Could you check a few things on this model? Use its own coordinates, in mm. A direction names the side the tool comes from. Coordinates: 2 decimals unless noted, no trailing zeros. Order: outer loops, then holes, each group sorted by start corner. A loop starts at its lowest first (then second) coordinate and runs counter-clockwise, first axis right, second up. Notation, with made-up numbers: (9, 71.5) -> (64, 71.5) arc R24 cw to (64, 109.5) -> close; hole circle Ø2 at (-18.5, 9). An arc over 180 degrees is marked (long way). Use a Markdown table: item, result. Add a question column.
1) If we section it at B-B (x = 54): Write out the boundary of the cut face in (y, z).
2) If we section it at D-D (z = -1): Write out the boundary of the cut face in (x, y).
3) If we section it at A-A (z = -6): Give the number of separate pieces and of enclosed holes in the cut face, plus the area to 3 significant figures.
4) Thinking about a two-plate mould opening in X: for faces 5 (the flat face through (43, 6, 0)), 6 (the cylindrical face through (26.11, 2.46, -7.34)), 7 (the cylindrical face through (21.804, 15.944, -6.488)), 8 (the flat face through (76, 6, -8)), which applies, +X half, -X half, draft (parallel to the pull), parting line (faces both ways), or undercut?
5) Which directions (+Z, -Z, +X, -X, +Y, -Y) give clear straight access to the entire face, cutting with the end or side of a thin tool? Please do faces 1 (the cylindrical face through (62.004, 15.944, -4.962)), 2 (the flat face through (24, 5, -8)), 3 (the cylindrical face through (59, 6, -11)), 4 (the cylindrical face through (22.513, 12.395, -5.805)).
6) Will these pins go through, and if not, where does the flat tip stop? pin 1 Ø4.5 at (x, z) = (64, -6) entering from -Y; pin 2 Ø3 at (x, y) = (53, 4.5) entering from -Z; pin 3 Ø3 at (x, z) = (59, -10) entering from +Y.
7) If we section it at C-C (y = 15): Write out the boundary of the cut face in (x, z).
8) If I drill on L1, parallel to X at y = 14.5, z = -6; L2, parallel to Y at x = 54, z = -9.75; L3, parallel to Y at x = 75.5, z = -1.5, over which ranges is the centre line in solid material (lowest first)? Write a range as [from, to].
```python
from build123d import *

# Parameters (mm, degrees)
BOSS_EXTRUDE1_DEPTH = 12
SKETCH2_R           = 2.5
CUT_EXTRUDE1_DEPTH  = 5
SKETCH3_R           = 1.5
CUT_EXTRUDE2_DEPTH  = 90.089842294
SKETCH4_R           = 2.25
SKETCH4_R_2         = 1.5
BOSS_EXTRUDE2_DEPTH = 8
SKETCH5_R           = 5
CUT_EXTRUDE3_DEPTH  = 3
SKETCH6_R           = 1.5
CUT_EXTRUDE4_DEPTH  = 91.691785736


with BuildPart() as part:
    # Sketch1 → Boss-Extrude1 (new body)
    with BuildSketch(Plane(origin=(0, 0, 0), x_dir=(1, 0, 0), z_dir=(0, 1, 0))):
        Polygon((0, 0), (88, 0), (88, 4), (64, 12), (24, 12), (0, 4), align=None)
    extrude(amount=BOSS_EXTRUDE1_DEPTH)

    # Sketch2 → Cut-Extrude1 (cut)
    with BuildSketch(Plane(origin=(0, 0, 0), x_dir=(-1, 0, 0), z_dir=(0, -1, 0))):
        with Locations(Location((-24, 6, 0), (0, 0, 90))):
            Circle(SKETCH2_R)
        with Locations(Location((-64, 6, 0), (0, 0, 90))):
            Circle(SKETCH2_R)
    extrude(amount=-CUT_EXTRUDE1_DEPTH, mode=Mode.SUBTRACT)

    # Sketch3 → Cut-Extrude2 (cut, through all)
    with BuildSketch(Plane(origin=(0, 5, 0), x_dir=(-1, 0, 0), z_dir=(0, -1, 0))):
        with Locations(Location((-24, 6, 0), (0, 0, 90))):
            Circle(SKETCH3_R)
        with Locations(Location((-64, 6, 0), (0, 0, 90))):
            Circle(SKETCH3_R)
    extrude(amount=-CUT_EXTRUDE2_DEPTH, mode=Mode.SUBTRACT)

    # Sketch4 → Boss-Extrude2 (add)
    with BuildSketch(Plane(origin=(0, 12, 0), x_dir=(1, 0, 0), z_dir=(0, 1, 0))):
        with Locations(Location((24, 6, 0), (0, 0, 270))):
            Circle(SKETCH4_R)
        with Locations(Location((24, 6, 0), (0, 0, 90))):
            Circle(SKETCH4_R_2, mode=Mode.SUBTRACT)
        with Locations(Location((64, 6, 0), (0, 0, 270))):
            Circle(SKETCH4_R)
        with Locations(Location((64, 6, 0), (0, 0, 90))):
            Circle(SKETCH4_R_2, mode=Mode.SUBTRACT)
    extrude(amount=BOSS_EXTRUDE2_DEPTH)

    # Sketch5 → Cut-Extrude3 (cut)
    with BuildSketch(Plane(origin=(0, 0, -12), x_dir=(-1, 0, 0), z_dir=(0, 0, -1))):
        with Locations((-54, 6)):
            Circle(SKETCH5_R)
    extrude(amount=-CUT_EXTRUDE3_DEPTH, mode=Mode.SUBTRACT)

    # Sketch6 → Cut-Extrude4 (cut, through all)
    with BuildSketch(Plane(origin=(0, 0, -9), x_dir=(-1, 0, 0), z_dir=(0, 0, -1))):
        with Locations((-54, 6)):
            Circle(SKETCH6_R)
    extrude(amount=-CUT_EXTRUDE4_DEPTH, mode=Mode.SUBTRACT)


solid = part.part
```
Answer sheet:
| question | item | result |
|---|---|---|
| 1 | outline | (0, -12) -> (1, -12) -> (1, -9) -> (4.5, -9) -> (4.5, 0) -> (0, 0) -> close; (7.5, -9) -> (11, -9) -> (11, -12) -> (12, -12) -> (12, 0) -> (7.5, 0) -> close |
| 2 | outline | (0, 0) -> (88, 0) -> (88, 12) -> (0, 12) -> close; hole circle Ø3 at (54, 6) |
| 3 | separate pieces | 3 |
| 3 | enclosed holes | 1 |
| 3 | area | 837 mm2 |
| 4 | face 5 | draft |
| 4 | face 6 | undercut |
| 4 | face 7 | undercut |
| 4 | face 8 | +X half |
| 5 | face 1 | +Y |
| 5 | face 2 | -Y |
| 5 | face 3 | -Z |
| 5 | face 4 | +Y, -Y |
| 6 | pin 1 | y = 5 |
| 6 | pin 2 | z = -9 |
| 6 | pin 3 | y = 12 |
| 7 | outline | circle Ø4.5 at (24, -6); circle Ø4.5 at (64, -6); hole circle Ø3 at (24, -6); hole circle Ø3 at (64, -6) |
| 8 | L1 | [21.75, 22.5], [25.5, 26.25], [61.75, 62.5], [65.5, 66.25] |
| 8 | L2 | [0, 1], [11, 12] |
| 8 | L3 | [0, 12] |
